from build123d import *

# Parameters (mm, degrees)
BOSS_EXTRUDE1_DEPTH       = 0.5
F_3_0MM_DOWEL_HOLE1_D     = 3
F_3_0MM_DOWEL_HOLE1_DEPTH = 12.75
F_3_0MM_DOWEL_HOLE1_TIP   = 0.901290929
M3_TAPPED_HOLE2_D         = 2.5
M3_TAPPED_HOLE2_DEPTH     = 7.5
M3_TAPPED_HOLE2_TIP       = 0.751075774


with BuildPart() as part:
    # Sketch1 → Boss-Extrude1 (new body)
    with BuildSketch(Plane(origin=(0, 0, 0), x_dir=(1, 0, 0), z_dir=(0, 1, 0))):
        Polygon((-0.59160691, 16.53307367), (-0.59160691, -3.46692633), (3.40839309, -3.46692633), (10.40839309, 4.53307367), (10.40839309, 6.53307367), (10.40839309, 8.53307367), (3.40839309, 16.53307367), align=None)
    extrude(amount=BOSS_EXTRUDE1_DEPTH)

    # Ø3.0mm Dowel Hole1
    with Locations(Plane(origin=(1.40839309, 0.5, -13.53307367), x_dir=(0, 0, 1), z_dir=(0, 1, 0))):
        with Locations((0, 0), (14, 0)):
            Hole(F_3_0MM_DOWEL_HOLE1_D / 2, depth=F_3_0MM_DOWEL_HOLE1_DEPTH)
            with Locations((0, 0, -(F_3_0MM_DOWEL_HOLE1_DEPTH + F_3_0MM_DOWEL_HOLE1_TIP / 2))):  # 118° drill point
                Cone(0, F_3_0MM_DOWEL_HOLE1_D / 2, F_3_0MM_DOWEL_HOLE1_TIP, mode=Mode.SUBTRACT)

    # M3 Tapped Hole2
    with Locations(Plane(origin=(7.034946216, 0, -6.53307367), x_dir=(0, 0, -1), z_dir=(0, -1, 0))):
        with Locations((0, 0)):
            Hole(M3_TAPPED_HOLE2_D / 2, depth=M3_TAPPED_HOLE2_DEPTH)
            with Locations((0, 0, -(M3_TAPPED_HOLE2_DEPTH + M3_TAPPED_HOLE2_TIP / 2))):  # 118° drill point
                Cone(0, M3_TAPPED_HOLE2_D / 2, M3_TAPPED_HOLE2_TIP, mode=Mode.SUBTRACT)


solid = part.part
The model under review builds one solid part; all positions refer to its coordinate system, in mm. Give positions to 0.01 mm unless a question says otherwise; leave off trailing zeros. Order: outer loops, then holes, each group sorted by start corner. A loop starts at its lowest first (then second) coordinate and runs counter-clockwise, first axis right, second up. Notation, with made-up numbers: M 28.25,83 L 57.25,83 A33 ccw 57.25,116 Z; hole C 1,21.25 d6. An arc over 180 degrees is marked long. Answer in a Markdown table with one row per item. Add a question column.
1. To check wall thickness, follow line 1 along X through (y, z) = (0.1, -6); line 2 along X through (y, z) = (0.15, -6.5); line 3 along Z through (x, y) = (7.5, 0.3). State the ranges of each line that lie inside material, in increasing order.
2. Add section D-D on z = 0.5. State the section outline as (x, y) points, plus the area to 3 significant figures.
3. Add section C-C on x = 0.75. State the section outline as (y, z) points, plus the area to 3 significant figures.
4. Add section A-A on z = -6.5. State the section outline as (x, y) points, plus the area to 3 significant figures.
5. For pin 1 Ø3 at (x, z) = (2, 1) entering from +Y, flat-tipped, find the tip position at first contact; note if it passes through.
6. Add section B-B on y = 0.1. State the section outline as (x, z) points, plus the area to 3 significant figures.
7. Mouldability with a two-part tool opening along X and no side actions: class faces 1 (the cylindrical face through (0.834, 0.246, -0.919)), 2 (the flat face through (6.957, 0.246, -12.477)), 3 (the flat face through (4, 0.5, -7)) as released by +X, released by -X, zero draft, split by the parting line, or undercut.
The answers:
| question | item | result |
|---|---|---|
| 1 | line 1 | -0.59 to 5.9, 8.17 to 10.41 |
| 1 | line 2 | -0.59 to 5.79, 8.28 to 10.41 |
| 1 | line 3 | -11.86 to -7.69, -5.37 to -1.21 |
| 2 | outline | M -0.59,0 L -0.09,0 L -0.09,0.5 L -0.59,0.5 Z; M 2.91,0 L 6,0 L 6,0.5 L 2.91,0.5 Z |
| 2 | area | 1.80 mm2 |
| 3 | outline | M 0,-16.53 L 0.5,-16.53 L 0.5,-14.88 L 0,-14.88 Z; M 0,-12.19 L 0.5,-12.19 L 0.5,-0.88 L 0,-0.88 Z; M 0,1.81 L 0.5,1.81 L 0.5,3.47 L 0,3.47 Z |
| 3 | area | 7.30 mm2 |
| 4 | outline | M -0.59,0 L 5.79,0 L 5.79,0.5 L -0.59,0.5 Z; M 8.28,0 L 10.41,0 L 10.41,0.5 L 8.28,0.5 Z |
| 4 | area | 4.25 mm2 |
| 5 | pin 1 | y = 0.5 |
| 6 | outline | M -0.59,-16.53 L 3.41,-16.53 L 10.41,-8.53 L 10.41,-4.53 L 3.41,3.47 L -0.59,3.47 Z; hole C 1.41,-13.53 d3; hole C 1.41,0.47 d3; hole C 7.03,-6.53 d2.5 |
| 6 | area | 145 mm2 |
| 7 | face 1 | undercut |
| 7 | face 2 | released by +X |
| 7 | face 3 | zero draft |
